```python
from build123d import *

# Parameters (mm, degrees)
CUT_EXTRUDE_1_REACH = 62
SKETCH_9_R          = 2.25
SKETCH_9_R_2        = 5
SKETCH_9_R_3        = 1.7
SKETCH_11_R         = 2.9
CUT_EXTRUDE_2_DEPTH = 10


with BuildPart() as part:
    # 草图1 → 旋转1 (revolve)
    with BuildSketch(Plane(origin=(0, 0, 0), x_dir=(1, 0, 0), z_dir=(0, 1, 0))):
        Polygon((38, -15), (25, -15), (25, -2), (23, 0), (0, 0), (0, -5), (20, -5), (20, -17), (23, -20), (40, -20), (40, -17), align=None)
    revolve(axis=Axis((0, 0, 0), (0, 0, 1)))

    # 草图9 → 切除-拉伸1 (cut, up to next)
    with BuildSketch(Plane(origin=(0, 0, 0), x_dir=(-1, 0, 0), z_dir=(0, 0, -1)), mode=Mode.PRIVATE) as cut_extrude_1_sk1:
        with Locations((-8.131727984, 8.131727984)):
            Circle(SKETCH_9_R)
    cut_extrude_1_tool1 = extrude(cut_extrude_1_sk1.sketch, amount=-CUT_EXTRUDE_1_REACH, mode=Mode.PRIVATE) & part.part
    # 草图9 → 切除-拉伸1 (cut, up to next)
    with BuildSketch(Plane(origin=(0, 0, 0), x_dir=(-1, 0, 0), z_dir=(0, 0, -1)), mode=Mode.PRIVATE) as cut_extrude_1_sk2:
        with Locations((8.131727984, 8.131727984)):
            Circle(SKETCH_9_R)
    cut_extrude_1_tool2 = extrude(cut_extrude_1_sk2.sketch, amount=-CUT_EXTRUDE_1_REACH, mode=Mode.PRIVATE) & part.part
    # 草图9 → 切除-拉伸1 (cut, up to next)
    with BuildSketch(Plane(origin=(0, 0, 0), x_dir=(-1, 0, 0), z_dir=(0, 0, -1)), mode=Mode.PRIVATE) as cut_extrude_1_sk3:
        with Locations((8.131727984, -8.131727984)):
            Circle(SKETCH_9_R)
    cut_extrude_1_tool3 = extrude(cut_extrude_1_sk3.sketch, amount=-CUT_EXTRUDE_1_REACH, mode=Mode.PRIVATE) & part.part
    # 草图9 → 切除-拉伸1 (cut, up to next)
    with BuildSketch(Plane(origin=(0, 0, 0), x_dir=(-1, 0, 0), z_dir=(0, 0, -1)), mode=Mode.PRIVATE) as cut_extrude_1_sk4:
        with Locations((-8.131727984, -8.131727984)):
            Circle(SKETCH_9_R)
    cut_extrude_1_tool4 = extrude(cut_extrude_1_sk4.sketch, amount=-CUT_EXTRUDE_1_REACH, mode=Mode.PRIVATE) & part.part
    # 草图9 → 切除-拉伸1 (cut, up to next)
    with BuildSketch(Plane(origin=(0, 0, 0), x_dir=(-1, 0, 0), z_dir=(0, 0, -1)), mode=Mode.PRIVATE) as cut_extrude_1_sk5:
        Circle(SKETCH_9_R_2)
    cut_extrude_1_tool5 = extrude(cut_extrude_1_sk5.sketch, amount=-CUT_EXTRUDE_1_REACH, mode=Mode.PRIVATE) & part.part
    # 草图9 → 切除-拉伸1 (cut, up to next)
    with BuildSketch(Plane(origin=(0, 0, 0), x_dir=(-1, 0, 0), z_dir=(0, 0, -1)), mode=Mode.PRIVATE) as cut_extrude_1_sk6:
        with Locations((0, 15.5)):
            Circle(SKETCH_9_R_3)
    cut_extrude_1_tool6 = extrude(cut_extrude_1_sk6.sketch, amount=-CUT_EXTRUDE_1_REACH, mode=Mode.PRIVATE) & part.part
    # 草图9 → 切除-拉伸1 (cut, up to next)
    with BuildSketch(Plane(origin=(0, 0, 0), x_dir=(-1, 0, 0), z_dir=(0, 0, -1)), mode=Mode.PRIVATE) as cut_extrude_1_sk7:
        with Locations((-15.5, 0)):
            Circle(SKETCH_9_R_3)
    cut_extrude_1_tool7 = extrude(cut_extrude_1_sk7.sketch, amount=-CUT_EXTRUDE_1_REACH, mode=Mode.PRIVATE) & part.part
    # 草图9 → 切除-拉伸1 (cut, up to next)
    with BuildSketch(Plane(origin=(0, 0, 0), x_dir=(-1, 0, 0), z_dir=(0, 0, -1)), mode=Mode.PRIVATE) as cut_extrude_1_sk8:
        with Locations((0, -15.5)):
            Circle(SKETCH_9_R_3)
    cut_extrude_1_tool8 = extrude(cut_extrude_1_sk8.sketch, amount=-CUT_EXTRUDE_1_REACH, mode=Mode.PRIVATE) & part.part
    # 草图9 → 切除-拉伸1 (cut, up to next)
    with BuildSketch(Plane(origin=(0, 0, 0), x_dir=(-1, 0, 0), z_dir=(0, 0, -1)), mode=Mode.PRIVATE) as cut_extrude_1_sk9:
        with Locations((15.5, 0)):
            Circle(SKETCH_9_R_3)
    cut_extrude_1_tool9 = extrude(cut_extrude_1_sk9.sketch, amount=-CUT_EXTRUDE_1_REACH, mode=Mode.PRIVATE) & part.part
    add(cut_extrude_1_tool1.solids().sort_by_distance((8.131728, 8.131728, 0))[0], mode=Mode.SUBTRACT)
    add(cut_extrude_1_tool2.solids().sort_by_distance((-8.131728, 8.131728, 0))[0], mode=Mode.SUBTRACT)
    add(cut_extrude_1_tool3.solids().sort_by_distance((-8.131728, -8.131728, 0))[0], mode=Mode.SUBTRACT)
    add(cut_extrude_1_tool4.solids().sort_by_distance((8.131728, -8.131728, 0))[0], mode=Mode.SUBTRACT)
    add(cut_extrude_1_tool5.solids().sort_by_distance((0, 0, 0))[0], mode=Mode.SUBTRACT)
    add(cut_extrude_1_tool6.solids().sort_by_distance((0, 15.5, 0))[0], mode=Mode.SUBTRACT)
    add(cut_extrude_1_tool7.solids().sort_by_distance((15.5, 0, 0))[0], mode=Mode.SUBTRACT)
    add(cut_extrude_1_tool8.solids().sort_by_distance((0, -15.5, 0))[0], mode=Mode.SUBTRACT)
    add(cut_extrude_1_tool9.solids().sort_by_distance((-15.5, 0, 0))[0], mode=Mode.SUBTRACT)

    # 草图11 → 切除-拉伸2 (cut)
    with BuildSketch(Plane.XY.offset(20)):
        with Locations((0, 35)):
            Circle(SKETCH_11_R)
        with Locations((-30.310889132, 17.5)):
            Circle(SKETCH_11_R)
        with Locations((-30.310889132, -17.5)):
            Circle(SKETCH_11_R)
        with Locations((0, -35)):
            Circle(SKETCH_11_R)
        with Locations((30.310889132, -17.5)):
            Circle(SKETCH_11_R)
        with Locations((30.310889132, 17.5)):
            Circle(SKETCH_11_R)
    extrude(amount=-CUT_EXTRUDE_2_DEPTH, mode=Mode.SUBTRACT)


solid = part.part
```
Check sheet for the modelled part. Datum: model origin and axes. Units: mm. A direction names the side the tool comes from. Round coordinates to 2 decimals unless told otherwise and drop trailing zeros. Order: outer loops, then holes, each group sorted by start corner. A loop starts at its lowest first (then second) coordinate and runs counter-clockwise, first axis right, second up.
1) Go/stop test with flat-tipped pins: pin 1 Ø10 at (y, z) = (-17, 3) entering from -X; pin 2 Ø1.5 at (y, z) = (11.5, 3) entering from -X; pin 3 Ø2 at (x, z) = (-21, 11) entering from -Y; pin 4 Ø4.5 at (x, y) = (0, -15.5) entering from -Z. Record where each tip stops, or that it passes through.
2) Mould release check, pull along X, two halves, no side actions. Record for faces 1 (the cylindrical face through (-8.67, -39.05, 18.48)), 2 (the cylindrical face through (28.01, -19.265, 17.535)), 3 (the flat face through (25, -8, 15)): +X half, -X half, draft (parallel to the pull), parting line (faces both ways), or undercut.
3) Scan lines: line 1 (Y direction, x = 0, z = 2.4); line 2 (Z direction, x = 28, y = 11); line 3 (X direction, y = 12, z = 9.5). Record each from-to range of solid material in increasing order.
4) Section check A-A (y = 0). Give the number of separate pieces and of enclosed holes in the cut face, and give its area (3 significant figures).
5) Tool access check on faces 4 (the cylindrical face through (28.01, 15.735, 17.535)), 5 (the flat face through (-4, -4, 5)). Record the directions out of +Z, -Z, +X, -X, +Y, -Y that give a thin tool (end or side, any length) a straight path to the whole face; none if there is none.
6) Section check B-B (z = 13.5). Record the boundary of the cut face in (x, y), and give its area (3 significant figures).
Result:
1. pin 1: stops at x = -21.93
1. pin 2: stops at x = -22.57
1. pin 3: stops at y = -15
1. pin 4: stops at z = 0
2. face 1: parting line
2. face 2: undercut
2. face 3: draft
3. line 1: y = -25 to -17.2, -13.8 to -5, 5 to 13.8, 17.2 to 25
3. line 2: z = 15 to 20
3. line 3: x = -21.93 to -16, 16 to 21.93
4. separate pieces: 4
4. enclosed holes: 0
4. area: 449 mm2
5. face 4: +Z, -Z
5. face 5: +Z
6. outline: circle Ø50 at (0, 0); hole circle Ø40 at (0, 0)
6. area: 707 mm2
